from build123d import *

# Parameters (mm, degrees)
BOSS_EXTRUDE1_DEPTH      = 17
BOSS_EXTRUDE1_DEPTH_BACK = 17
BOSS_EXTRUDE2_DEPTH      = 6
BOSS_EXTRUDE2_DEPTH_BACK = 6
SKETCH1_3_R              = 4
SKETCH2_R                = 2.5
CUT_EXTRUDE1_DEPTH       = 45.955533586


with BuildPart() as part:
    # Sketch1 → Boss-Extrude1 (new, two sides: drawn at the far end of the back side and taken through both)
    with BuildSketch(Plane(origin=(0, 0, 0), x_dir=(1, 0, 0), z_dir=(0, 1, 0)).offset(-BOSS_EXTRUDE1_DEPTH_BACK)):
        with BuildLine():
            Line((22, -7), (22, -12))
            ThreePointArc((22, -12), (30.485281374, -8.485281374), (34, 0))
            ThreePointArc((34, 0), (30.485281374, 8.485281374), (22, 12))
            Line((22, 12), (22, 7))
            ThreePointArc((22, 7), (29, 0), (22, -7))
        make_face()
        with BuildLine():
            ThreePointArc((22, 12), (10, 0), (22, -12))
            Line((22, -12), (22, -7))
            ThreePointArc((22, -7), (18.031373033, -5.766281297), (15.461651585, -2.5))
            Line((15.461651585, -2.5), (13, -2.5))
            Line((13, -2.5), (13, 2.5))
            Line((13, 2.5), (15.461651585, 2.5))
            ThreePointArc((15.461651585, 2.5), (18.031373033, 5.766281297), (22, 7))
            Line((22, 7), (22, 12))
        make_face()
    extrude(amount=BOSS_EXTRUDE1_DEPTH + BOSS_EXTRUDE1_DEPTH_BACK)

    # Sketch1_3 → Boss-Extrude2 (add, two sides: drawn at the far end of the back side and taken through both)
    with BuildSketch(Plane(origin=(0, 0, 0), x_dir=(1, 0, 0), z_dir=(0, 1, 0)).offset(-BOSS_EXTRUDE2_DEPTH_BACK)):
        with BuildLine():
            Line((-22, -7), (-22, -12))
            Line((-22, -12), (22, -12))
            ThreePointArc((22, -12), (10, 0), (22, 12))
            Line((22, 12), (-22, 12))
            Line((-22, 12), (-22, 7))
            Line((-22, 7), (-10, 7))
            Line((-10, 7), (-10, -7))
            Line((-10, -7), (-22, -7))
        make_face()
        with Locations(Location((-2, 0, 0), (0, 0, 270))):
            Circle(SKETCH1_3_R, mode=Mode.SUBTRACT)
    extrude(amount=BOSS_EXTRUDE2_DEPTH + BOSS_EXTRUDE2_DEPTH_BACK)

    # Sketch2 → Cut-Extrude1 (cut, through all)
    with BuildSketch(Plane.XY.offset(12)):
        with BuildLine():
            Line((-16, 6), (-22, 6))
            Line((-22, 6), (-22, -5e-09))
            ThreePointArc((-22, -5e-09), (-20.242640689, 4.242640685), (-16, 6))
        make_face()
        with BuildLine():
            ThreePointArc((-16, -6), (-20.242640685, -4.242640689), (-22, -5e-09))
            Line((-22, -5e-09), (-22, -6))
            Line((-22, -6), (-16, -6))
        make_face()
        with Locations((-16, 0)):
            Circle(SKETCH2_R)
    extrude(amount=-CUT_EXTRUDE1_DEPTH, mode=Mode.SUBTRACT)


solid = part.part
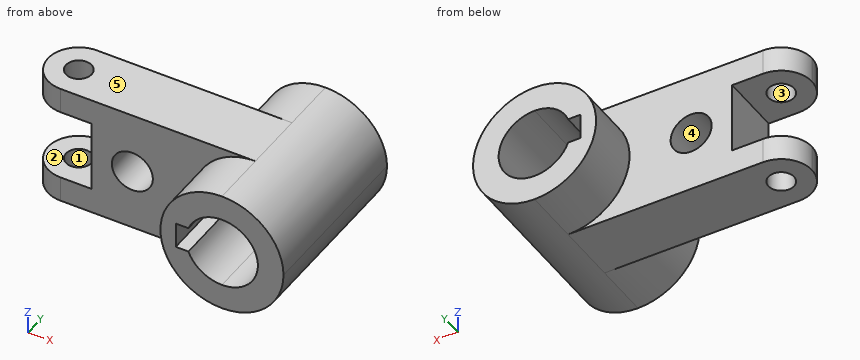
Design review of the part built by this model. Coordinates are the model's own, in mm. Face numbers are marked on the shaded views. A direction names the side the tool comes from. Coordinates: 2 decimals unless noted, no trailing zeros. Order: outer loops, then holes, each group sorted by start corner. A loop starts at its lowest first (then second) coordinate and runs counter-clockwise, first axis right, second up.
Item 1: Take a section at D-D, the plane x = -17.5. Write out the cut boundary in (y, z), then the cut area to 3 significant figures.
Item 2: Take a section at B-B, the plane z = -3.25. Write out the cut boundary in (x, y).
Item 3: For pin 1 Ø13 at (y, z) = (-0.5, 0) entering from -X; pin 2 Ø10.5 at (x, z) = (-2, 0) entering from -Y, all flat-tipped, find the tip position at first contact; note any pin that passes through.
Item 4: Take a section at A-A, the plane x = -2. Write out the cut boundary in (y, z), then the cut area to 3 significant figures.
Item 5: For line 1 (X direction, y = 2.25, z = 0); line 2 (Y direction, x = -16, z = -9.9); line 3 (Z direction, x = 15, y = 2), list the stretches that pass through material, from the lowest coordinate up.
Item 6: For the marked faces 1 and 2, list the 3-axis set-ups (+Z, -Z, +X, -X, +Y, -Y) from which the entire face can be reached by the end or side of a thin tool; tool diameter is ignored.
Item 7: The part is to be moulded in two halves that separate along Z. For the marked faces 3, 4 and 5, say which applies: pulls with the +Z half, pulls with the -Z half, needs draft (parallel to the pull), parting line crosses it, or undercut.
Item 8: Take a section at C-C, the plane y = -1.5. Write out the cut boundary in (x, z).
The answers:
1. outline: (-5.81, -12) - (-2, -12) - (-2, -7) - (-5.81, -7) - close; (-5.81, 7) - (-2, 7) - (-2, 12) - (-5.81, 12) - close; (2, -12) - (5.81, -12) - (5.81, -7) - (2, -7) - close; (2, 7) - (5.81, 7) - (5.81, 12) - (2, 12) - close
1. area: 76.2 mm2
2. outline: (-10, -6) - (-4.33, -6) - (-4.33, 6) - (-10, 6) - close; (0.33, -6) - (10.45, -6) - (10.45, -17) - (15.8, -17) - (15.8, 17) - (10.45, 17) - (10.45, 6) - (0.33, 6) - close; (28.2, -17) - (33.55, -17) - (33.55, 17) - (28.2, 17) - close
3. pin 1: stops at x = -10
3. pin 2: stops at y = -6
4. outline: (-6, -12) - (6, -12) - (6, -4) - (-6, -4) - close; (-6, 4) - (6, 4) - (6, 12) - (-6, 12) - close
4. area: 192 mm2
5. line 1: x = -10 to -6, 2 to 13, 29 to 34
5. line 2: y = -6 to -2.5, 2.5 to 6
5. line 3: z = -12 to -2.5, 2.5 to 12
6. face 1: +Z, -Z
6. face 2: -X, +Y, -Y
7. face 3: needs draft
7. face 4: undercut
7. face 5: pulls with the +Z half
8. outline: (-21.81, -12) - (-18, -12) - (-18, -7) - (-21.81, -7) - close; (-21.81, 7) - (-18, 7) - (-18, 12) - (-21.81, 12) - close; (-14, -12) - (22, -12) arc R12 ccw to (22, 12) - (-14, 12) - (-14, 7) - (-10, 7) - (-10, -7) - (-14, -7) - close; hole circle Ø8 at (-2, 0); hole (13, -2.5) - (15.46, -2.5) arc R7 ccw (long way) to (15.46, 2.5) - (13, 2.5) - close
